Could you check a few things on this model? Use its own coordinates, in mm. Face numbers are marked on the shaded views. Give positions to 0.01 mm unless a question says otherwise; leave off trailing zeros. Loops run counter-clockwise (first coordinate to the right, second up) from the corner with the lowest first, then second, coordinate; pieces in that order, holes last. Notation, with made-up numbers: M -19.75,53.25 L 1.25,53.25 A25 cw 1.25,75.25 Z; hole C -0.75,80 d6. An arc over 180 degrees is marked long. Answer in a Markdown table with one row per item. Add a question column.
1. I need wall thicknesses on line 1 along X through (y, z) = (8.25, 0.65); line 2 along X through (y, z) = (8.75, 1.1); line 3 along X through (y, z) = (-3.5, 0.65). Which ranges of each line are inside material? Lowest first, please. Write a range as from..to.
2. If we section it at B-B on z = 0.25: List the corners of the cut face in (x, y) for me, then the cut area to 3 significant figures.
3. If we section it at C-C on y = -1.75: List the corners of the cut face in (x, z) for me.
4. If we section it at D-D on x = 0: List the corners of the cut face in (y, z) for me, then the cut area to 3 significant figures.
5. If we section it at A-A on x = -9.75: List the corners of the cut face in (y, z) for me, then the cut area to 3 significant figures.
6. Thinking about a two-plate mould opening in Y: for the marked faces 1 and 2, which applies, released by +Y, released by -Y, zero draft, split by the parting line, or undercut?
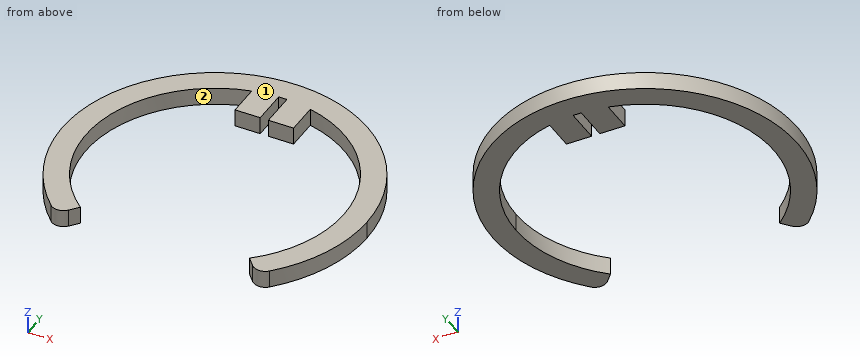
```python
from build123d import *

# Parameters (mm, degrees)
F1_DEPTH = 1.5
F2_R     = 1


with BuildPart() as f1:
    # F0 (on Top) → F1 (new body)
    with BuildSketch(Plane.XY):
        with BuildLine():
            ThreePointArc((2.5, 10.7121426428), (8.6168439698, 6.8373971656), (11, 0))
            ThreePointArc((11, 0), (10.0302093156, -4.5160714217), (7.2918361662, -8.2358439352))
            Line((7.2918361662, -8.2358439352), (8.61762456, -9.7332701053))
            ThreePointArc((8.61762456, -9.7332701053), (11.8538837366, -5.3371753166), (13, 0))
            ThreePointArc((13, 0), (-5.5098347525, 11.7746219048), (-8.3294955385, -9.9809570721))
            Line((-8.3294955385, -9.9809570721), (-7.0480346864, -8.4454252148))
            ThreePointArc((-7.0480346864, -8.4454252148), (-10.7025390982, 2.5407984674), (-2.5, 10.7121426428))
            ThreePointArc((-2.5, 10.7121426428), (-1.4319729731, 10.9063950692), (-0.35, 10.9944304082))
            ThreePointArc((-0.35, 10.9944304082), (0, 11), (0.35, 10.9944304082))
            ThreePointArc((0.35, 10.9944304082), (1.4319729731, 10.9063950692), (2.5, 10.7121426428))
        make_face()
        with BuildLine():
            Line((-0.35, 7.9944304082), (-0.35, 10.9944304082))
            ThreePointArc((-0.35, 10.9944304082), (-1.4319729731, 10.9063950692), (-2.5, 10.7121426428))
            Line((-2.5, 10.7121426428), (-2.5, 7.9944304082))
            Line((-2.5, 7.9944304082), (-0.35, 7.9944304082))
        make_face()
        with BuildLine():
            Line((2.5, 7.9944304082), (2.5, 10.7121426428))
            ThreePointArc((2.5, 10.7121426428), (1.4319729731, 10.9063950692), (0.35, 10.9944304082))
            Line((0.35, 10.9944304082), (0.35, 7.9944304082))
            Line((0.35, 7.9944304082), (2.5, 7.9944304082))
        make_face()
    extrude(amount=F1_DEPTH)

    # F2
    f2_edges = [f1.edges().sort_by_distance(p)[0] for p in [
        (-8.329496, -9.980957, 0.75),
        (8.617625, -9.73327, 0.75),
    ]]
    fillet(f2_edges, radius=F2_R)


solid = f1.part
```
Results:
| question | item | result |
|---|---|---|
| 1 | line 1 | -10.05..-7.28, -2.5..-0.35, 0.35..2.5, 7.28..10.05 |
| 1 | line 2 | -9.61..-6.67, -2.5..-0.35, 0.35..2.5, 6.67..9.61 |
| 1 | line 3 | -12.52..-10.43, 10.43..12.52 |
| 2 | outline | M -9.13,-9.25 A1 ccw -7.66,-9.18 L -7.05,-8.45 A11 cw -2.5,10.71 L -2.5,7.99 L -0.35,7.99 L -0.35,10.99 A11 cw 0.35,10.99 L 0.35,7.99 L 2.5,7.99 L 2.5,10.71 A11 cw 7.29,-8.24 L 7.93,-8.95 A1 ccw 9.4,-8.98 A13 ccw long Z |
| 2 | area | 129 mm2 |
| 3 | outline | M -12.88,0 L -10.86,0 L -10.86,1.5 L -12.88,1.5 Z; M 10.86,0 L 12.88,0 L 12.88,1.5 L 10.86,1.5 Z |
| 4 | outline | M 11,0 L 13,0 L 13,1.5 L 11,1.5 Z |
| 4 | area | 3.00 mm2 |
| 5 | outline | M -8.6,0 L -5.09,0 L -5.09,1.5 L -8.6,1.5 Z; M 5.09,0 L 8.6,0 L 8.6,1.5 L 5.09,1.5 Z |
| 5 | area | 10.5 mm2 |
| 6 | face 1 | zero draft |
| 6 | face 2 | undercut |
